```python
from build123d import *

# Parameters (mm, degrees)
F1_DEPTH  = 30
F2_R      = 25
F3_DEPTH  = 54
F4_W      = 50
F4_H      = 24
F5_DEPTH  = 21
F6_W      = 25
F6_H      = 50
F7_DEPTH  = 38
F8_W      = 30
F8_H      = 9
F11_W     = 16
F11_H     = 8
F12_DEPTH = 90.001


# Not quite as in the source:
# - a pattern or mirror of a feature is missing from the dataset's text; its kind, count and spacing are read off the source's solid


with BuildPart() as f1:
    # F0 (on Right) → F1 (new body, symmetric)
    with BuildSketch(Plane.YZ):
        Polygon((-45, 0), (0, 0), (45, 0), (45, 8), (25, 32), (0, 32), (-25, 32), (-45, 8), align=None)
    extrude(amount=F1_DEPTH, both=True)

    # F2 (on face) → F3 (join)
    with BuildSketch(Plane.XY.offset(32)):
        Circle(F2_R)
    extrude(amount=F3_DEPTH)

    # F4 (on face) → F5 (cut)
    with BuildSketch(Plane.XY.offset(86)):
        Rectangle(F4_W, F4_H)
    extrude(amount=-F5_DEPTH, mode=Mode.SUBTRACT)

    # F6 (on face) → F7 (cut)
    with BuildSketch(Plane.XY.offset(86)):
        with Locations((22.5, 0)):
            Rectangle(F6_W, F6_H)
    f7 = extrude(amount=-F7_DEPTH, mode=Mode.SUBTRACT)

    # F7_copies: F7 across plane
    add(f7.mirror(Plane(origin=(0, 0, 0), x_dir=(0, 0, -1), z_dir=(-1, 0, 0))), mode=Mode.SUBTRACT)

    # F10: sweep along a path in F9
    with BuildLine(Plane.YZ.offset(30)) as f10_path:
        Line((-35, 20), (51.1633306742, 20))
    # F8 (on face) → F10 (sweep, cut)
    with BuildSketch(Plane(origin=(0, -30.4918032787, 25.4098360656), x_dir=(1, 0, 0), z_dir=(0, -0.7682212796, 0.6401843997))):
        with Locations((0, -4.9215290445)):
            Rectangle(F8_W, F8_H)
    sweep(path=f10_path.line, mode=Mode.SUBTRACT)

    # F11 (on face) → F12 (cut, through all)
    with BuildSketch(Plane.XZ.offset(45)):
        with Locations((0, 4)):
            Rectangle(F11_W, F11_H)
    extrude(amount=-F12_DEPTH, mode=Mode.SUBTRACT)


solid = f1.part
```
For this review, take the finished solid that the model builds, in its own axes (mm). A direction names the side the tool comes from. Round coordinates to 2 decimals unless told otherwise and drop trailing zeros. Write each loop counter-clockwise with the first axis right and the second up, starting at its lowest first coordinate (ties: lowest second). Pieces come first, ordered by that corner, then holes. Notation, with made-up numbers: (84, 47.5) -> (137, 47.5) arc R23 cw to (137, 74.5) -> close; hole circle Ø8 at (51, -39). An arc over 180 degrees is marked (long way). One line per question, with ' | ' between items. Start each with the question number.
1) Add section B-B (z = 19.5). Write out the cut boundary in (x, y).
2) Mouldability with a two-part tool opening along Y and no side actions: class faces 1 (the flat face through (0, -12, 76)), 2 (the flat face through (0, 12, 76)), 3 (the flat face through (-19, -45, 4)), 4 (the flat face through (30, -1, 13)) as +Y half, -Y half, draft (parallel to the pull), parting line (faces both ways), or undercut.
3) For pin 1 Ø15 at (x, y) = (18.5, -4) entering from +Z; pin 2 Ø10 at (x, z) = (-2, 73) entering from -Y; pin 3 Ø15 at (x, y) = (-16, 7) entering from +Z, all flat-tipped, find the tip position at first contact; note any pin that passes through.
4) Add section A-A (y = -28.5). Write out the cut boundary in (x, z).
5) Add section D-D (y = 0). Write out the cut boundary in (x, z), and give its area (3 significant figures).
6) Machinability: for faces 5 (the flat face through (26, -2, 32)), 6 (the flat face through (-26, -2, 32)), 7 (the flat face through (8, -1, 4)), 8 (the flat face through (0, 0, 65)), 9 (the flat face through (15, -1, 20)), which of the approach directions +Z, -Z, +X, -X, +Y, -Y give a long, thin tool a straight path to every point of the face, cutting with its end or side? Answer none if there is none.
7) Wall thickness on line 1 along Z through (x, y) = (-2.5, -13.5); line 2 along Z through (x, y) = (11.5, -19); line 3 along X through (y, z) = (-22, 6): over which ranges is each line inside the solid? List them lowest first.
8) Add section C-C (x = 4). Write out the cut boundary in (y, z), and give its area (3 significant figures).
Reported:
1) outline: (-30, -35.42) -> (-15, -35.42) -> (-15, 35.42) -> (-30, 35.42) -> close; (15, -35.42) -> (30, -35.42) -> (30, 35.42) -> (15, 35.42) -> close
2) face 1: undercut | face 2: undercut | face 3: -Y half | face 4: draft
3) pin 1: stops at z = 48 | pin 2: stops at y = -25 | pin 3: stops at z = 65
4) outline: (-30, 0) -> (-8, 0) -> (-8, 8) -> (8, 8) -> (8, 0) -> (30, 0) -> (30, 27.8) -> (-30, 27.8) -> close; hole (-15, 18.17) -> (15, 18.17) -> (15, 25.09) -> (-15, 25.09) -> close
5) outline: (-30, 0) -> (-8, 0) -> (-8, 8) -> (8, 8) -> (8, 0) -> (30, 0) -> (30, 32) -> (25, 32) -> (25, 48) -> (10, 48) -> (10, 65) -> (-10, 65) -> (-10, 48) -> (-25, 48) -> (-25, 32) -> (-30, 32) -> close; hole (-15, 18.17) -> (15, 18.17) -> (15, 25.09) -> (-15, 25.09) -> close | area: 2,720 mm²
6) face 5: +Z, +X | face 6: +Z, -X | face 7: -Z, +Y, -Y | face 8: +Z, +X, -X | face 9: +Y, -Y
7) line 1: z = 8 to 18.17, 25.09 to 86 | line 2: z = 0 to 18.17, 25.09 to 48 | line 3: x = -30 to -8, 8 to 30
8) outline: (-45, 8) -> (45, 8) -> (36.52, 18.17) -> (-36.52, 18.17) -> close; (-30.76, 25.09) -> (30.76, 25.09) -> (25, 32) -> (24.68, 32) -> (24.68, 86) -> (12, 86) -> (12, 65) -> (-12, 65) -> (-12, 86) -> (-24.68, 86) -> (-24.68, 32) -> (-25, 32) -> close | area: 3,380 mm²
